Autodesk Inventor part; units mm, degrees
ref_plane "YZ Plane" through (0, 0, 0) normal (1, 0, 0) x (0, 1, 0)
ref_plane "XZ Plane" through (0, 0, 0) normal (0, 1, 0) x (-1, 0, 0)
ref_plane "XY Plane" through (0, 0, 0) normal (0, 0, 1) x (1, 0, 0)
sketch "Sketch1" plane through (0, 0, 0) normal (0, 1, 0) x (-1, 0, 0)
  line L0 (0, 0) -> (35, 0)
  line L1 (35, 0) -> (35, -30)
  line L2 (35, -30) -> (0, -30)
  line L3 (0, -30) -> (0, 0)
  circle A0 centre (30, -9.5) radius 2.5
  circle A1 centre (30, -20.5) radius 2.5
  line L4 (30, -9.5) -> (30, -20.5) construction
  circle A2 centre (8, -15) radius 2.75
  point P0 (35, -15)
  point P1 (30, -15)
  point P2 (0, -15)
  dimension "d0" = 30
  dimension "d1" = 35
  dimension "d2" = 5
  dimension "d3" = 5
  dimension "d4" = 11
  dimension "d5" = 5
  dimension "d6" = 5.5
  dimension "d7" = 8
extrude "Extrusion1" add sketch "Sketch1" along normal blind 2
fillet "Fillet1" radius 2 4 edges at (0, 1, -30) (0, 1, 0) (-35, 1, 0) (-35, 1, -30)
equation "\"d3\" = d2"
Work out the finished part from the listing and answer in its coordinate system (mm). Coordinates: 2 decimals unless noted, no trailing zeros. Loops run counter-clockwise (first coordinate to the right, second up) from the corner with the lowest first, then second, coordinate; pieces in that order, holes last. Notation, with made-up numbers: M 32.5,-6.75 L 37.5,-6.75 A24 cw 37.5,29.25 Z; hole C 74.5,8 d3. An arc over 180 degrees is marked long. Answer in a Markdown table with one row per item. Add a question column.
1. Consider L1, parallel to Z at x = -30, y = 0.75; L2, parallel to Z at x = -32, y = 1.45; L3, parallel to Z at x = -8, y = 0.75. Determine where each line is inside the solid, lowest interval first.
2. Find section D-D, the plane y = 1.7. Write down the section's boundary in (x, z), then the cut area to 3 significant figures.
3. Find section A-A, the plane z = -9.5. Write down the section's boundary in (x, y).
4. The mould has two halves that part along Z. Classify faces 1 (the cylindrical face through (-34.43, 1.01, -0.6)), 2 (the cylindrical face through (-30, 1, -23)), 3 (the flat face through (-17, 0, -15)): pulls with the +Z half, pulls with the -Z half, needs draft (parallel to the pull), parting line crosses it, or undercut.
5. Find section B-B, the plane x = -8. Write down the section's boundary in (y, z).
6. Find section C-C, the plane x = -30. Write down the section's boundary in (y, z).
Reported:
| question | item | result |
|---|---|---|
| 1 | L1 | z = -30 to -23, -18 to -12, -7 to 0 |
| 1 | L2 | z = -30 to -22, -19 to -11, -8 to 0 |
| 1 | L3 | z = -30 to -17.75, -12.25 to 0 |
| 2 | outline | M -35,-28 A2 ccw -33,-30 L -2,-30 A2 ccw 0,-28 L 0,-2 A2 ccw -2,0 L -33,0 A2 ccw -35,-2 Z; hole C -30,-20.5 d5; hole C -30,-9.5 d5; hole C -8,-15 d5.5 |
| 2 | area | 984 mm^2 |
| 3 | outline | M -35,0 L -32.5,0 L -32.5,2 L -35,2 Z; M -27.5,0 L 0,0 L 0,2 L -27.5,2 Z |
| 4 | face 1 | pulls with the +Z half |
| 4 | face 2 | undercut |
| 4 | face 3 | needs draft |
| 5 | outline | M 0,-30 L 2,-30 L 2,-17.75 L 0,-17.75 Z; M 0,-12.25 L 2,-12.25 L 2,0 L 0,0 Z |
| 6 | outline | M 0,-30 L 2,-30 L 2,-23 L 0,-23 Z; M 0,-18 L 2,-18 L 2,-12 L 0,-12 Z; M 0,-7 L 2,-7 L 2,0 L 0,0 Z |
